```python
from build123d import *

# Parameters (mm, degrees)
BOSS_EXTRUDE1_DEPTH = 50
CUT_EXTRUDE2_DEPTH  = 30
CUT_EXTRUDE3_DEPTH  = 15
BOSS_EXTRUDE4_DEPTH = 15
BOSS_EXTRUDE6_DEPTH = 52
BOSS_EXTRUDE7_DEPTH = 52
CUT_EXTRUDE6_DEPTH  = 52
BOSS_EXTRUDE8_DEPTH = 30
BOSS_EXTRUDE9_DEPTH = 15
CUT_EXTRUDE7_DEPTH  = 15
CUT_EXTRUDE8_DEPTH  = 15


with BuildPart() as part:
    # Sketch1 → Boss-Extrude1 (new body)
    with BuildSketch(Plane.XY):
        Polygon((0, 0), (0, 30), (20, 50), (70, 50), (70, 15), (55, 0), align=None)
    extrude(amount=BOSS_EXTRUDE1_DEPTH)

    # Sketch2 → Cut-Extrude2 (cut)
    with BuildSketch(Plane.XY.offset(50)):
        Polygon((0, 0), (50, 50), (20, 50), (0, 30), align=None)
    extrude(amount=-CUT_EXTRUDE2_DEPTH, mode=Mode.SUBTRACT)

    # Sketch4 → Cut-Extrude3 (cut)
    with BuildSketch(Plane(origin=(0, 0, 0), x_dir=(-1, 0, 0), z_dir=(0, 0, -1))):
        Polygon((-70, 15), (-55, 15), (-55, 0), align=None)
    extrude(amount=-CUT_EXTRUDE3_DEPTH, mode=Mode.SUBTRACT)

    # Sketch7 → Boss-Extrude4 (add)
    with BuildSketch(Plane(origin=(13.333333333, -13.333333333, -13.333333333), x_dir=(-0.816496581, -0.40824829, -0.40824829), z_dir=(0.577350269, -0.577350269, -0.577350269))):
        Polygon((-51.031036308, -10.606601718), (-69.402209379, 0), (-51.031036308, 10.606601718), align=None)
    extrude(amount=-BOSS_EXTRUDE4_DEPTH)

    # Sketch11 → Boss-Extrude6 (add)
    with BuildSketch(Plane.ZY):
        Polygon((20, 30), (50, 0), (20, 0), align=None)
    extrude(amount=-BOSS_EXTRUDE6_DEPTH)

    # Sketch12 → Boss-Extrude7 (add)
    with BuildSketch(Plane(origin=(0, 50, 0), x_dir=(1, 0, 0), z_dir=(0, 1, 0))):
        Polygon((20, -20), (50, -50), (50, -20), align=None)
    extrude(amount=-BOSS_EXTRUDE7_DEPTH)

    # Sketch13 → Cut-Extrude6 (cut)
    with BuildSketch(Plane.XZ):
        Polygon((20, 20), (50, 20), (50, 50), align=None)
    extrude(amount=CUT_EXTRUDE6_DEPTH, mode=Mode.SUBTRACT)

    # Sketch14 → Boss-Extrude8 (add)
    with BuildSketch(Plane(origin=(-16.666666667, 16.666666667, 16.666666667), x_dir=(-0.816496581, -0.40824829, -0.40824829), z_dir=(0.577350269, -0.577350269, -0.577350269))):
        Polygon((-20.412414523, 7.071067812), (-44.907311951, 21.213203436), (-81.649658093, 0), align=None)
    extrude(amount=BOSS_EXTRUDE8_DEPTH)

    # Sketch15 → Boss-Extrude9 (add)
    with BuildSketch(Plane(origin=(-16.666666667, 16.666666667, 16.666666667), x_dir=(0.816496581, 0.40824829, 0.40824829), z_dir=(-0.577350269, 0.577350269, 0.577350269))):
        Polygon((20.412414523, -35.355339059), (81.649658093, 0), (20.412414523, 7.071067812), align=None)
    extrude(amount=-BOSS_EXTRUDE9_DEPTH)

    # Sketch16 → Cut-Extrude7 (cut)
    with BuildSketch(Plane.XZ):
        Polygon((0, 50), (8.660254038, 32.679491924), (17.320508076, 41.339745962), align=None)
    extrude(amount=CUT_EXTRUDE7_DEPTH, mode=Mode.SUBTRACT)

    # Sketch17 → Cut-Extrude8 (cut)
    with BuildSketch(Plane(origin=(0, 0, 0), x_dir=(-1, 0, 0), z_dir=(0, -1, 0))):
        Polygon((0, 0), (-20, -20), (-20, 0), align=None)
    extrude(amount=-CUT_EXTRUDE8_DEPTH, mode=Mode.SUBTRACT)


solid = part.part
```
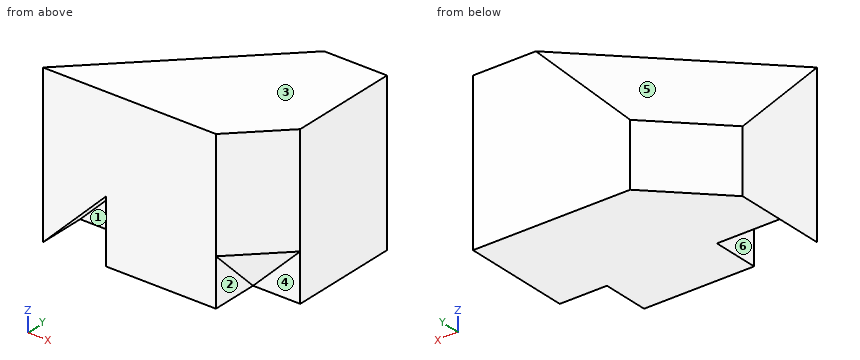
Here's how the part is built. I have some questions about the finished solid (model axes, mm). Face numbers are marked on the shaded views. A direction names the side the tool comes from. Coordinates: 2 decimals unless noted, no trailing zeros. Loops run counter-clockwise (first coordinate to the right, second up) from the corner with the lowest first, then second, coordinate; pieces in that order, holes last. Notation, with made-up numbers: (25.5, -39) - (65.5, -39) arc R31 ccw to (65.5, -1) - close; hole circle Ø6 at (-34.75, -13). An arc over 180 degrees is marked (long way). Return JSON: item names as keys, results as strings. Group by question number.
Item 1: I need wall thicknesses on line 1 (X direction, y = 9, z = 18); line 2 (Z direction, x = 9, y = 29); line 3 (Y direction, x = 58.5, z = 46.5). Which ranges of each line are inside material? Lowest first, please. Write a range as from..to.
Item 2: If we section it at C-C on z = 30.5: Write out the boundary of the cut face in (x, y), and give its area (3 significant figures).
Item 3: On a 3-axis mill with a long thin cutter (end or side, diameter ignored), from which of +Z, -Z, +X, -X, +Y, -Y can I reach the whole of each face in a straight line? I mean the marked faces 1, 2 and 3. Say none if no direction works.
Item 4: If we section it at A-A on y = 6.5: Write out the boundary of the cut face in (x, z).
Item 5: We'd pull the mould along X, two halves only. Please class the marked faces 4, 5 and 6: +X half, -X half, draft (parallel to the pull), parting line (faces both ways), or undercut.
Item 6: Will these pins go through, and if not, where does the flat tip stop? P1, Ø2, axis at y = 29.5, z = 31.5, coming from the -X side; P2, Ø12, axis at x = 63.5, z = 10.5, coming from the -Y side.
Item 7: If we section it at D-D on x = 59: Write out the boundary of the cut face in (y, z).
Item 8: If we section it at B-B on x = 5.5: Write out the boundary of the cut face in (y, z), and give its area (3 significant figures).
Calculated:
{
 "1": {"line 1": "x = 0..18, 20..64", "line 2": "z = 0..30", "line 3": "y = 3.5..50"},
 "2": {"outline": "(0, 0) - (55, 0) - (70, 15) - (70, 50) - (30.5, 50) - (0, 19.5) - close", "area": "2,920 mm^2"},
 "3": {"face 1": "-Z, -Y", "face 2": "-Z, +X, -Y", "face 3": "+Z, +X, -X, +Y, -Y"},
 "4": {"outline": "(0, 0) - (20, 20) - (20, 0) - (55, 0) - (55, 8.5) - (61.5, 15) - (61.5, 50) - (6.5, 50) - (0, 43.5) - close"},
 "5": {"face 4": "draft", "face 5": "-X half", "face 6": "undercut"},
 "6": {"P1": "stops at x = 9.59", "P2": "stops at y = 4.51"},
 "7": {"outline": "(4, 15) - (15, 4) - (15, 0) - (50, 0) - (50, 50) - (4, 50) - close"},
 "8": {"outline": "(0, 5.5) - (15, 5.5) - (15, 0) - (35.5, 0) - (35.5, 20) - (5.5, 50) - (0, 50) - close", "area": "1,240 mm^2"}
}
